Check sheet for the drawn part. Datum: minimum x, y, z corner. Units: mm. A direction names the side the tool comes from. Coordinates: 2 decimals unless noted, no trailing zeros. Order: outer loops, then holes, each group sorted by start corner. A loop starts at its lowest first (then second) coordinate and runs counter-clockwise, first axis right, second up. Notation, with made-up numbers: (73.5, -29) - (114.5, -29) arc R24 ccw to (114.5, -14) - close; hole circle Ø3 at (53.5, 34.5). An arc over 180 degrees is marked (long way). Return JSON: item names as keys, results as strings. Group by question number.
Item 1: Section check D-D on z = 38.5. Enter the section's corners in (x, y), then the cut area to 3 significant figures.
Item 2: Scan lines: probe 1 along Z at (x, y) = (3, 16.25); probe 2 along Y at (x, z) = (13, 127.5); probe 3 along X at (y, z) = (8.75, 122). Record each from-to range of solid material in increasing order.
Item 3: Section check C-C on z = 147. Enter the section's corners in (x, y).
Item 4: Tool access check on the marked faces 1, 2 and 3. Record the directions out of +Z, -Z, +X, -X, +Y, -Y that give a thin tool (end or side, any length) a straight path to the whole face; none if there is none.
Item 5: Section check A-A on x = 13. Enter the section's corners in (y, z).
Item 6: Gauge pin test, flat ends, axial feed: pin 1 (8 mm diameter, centred on x = 6, z = 137, fed in from -Y); pin 2 (12 mm diameter, centred on x = 11, z = 179.5, fed in from -Y); pin 3 (3 mm diameter, centred on x = 7, z = 144, fed in from +Y). Record the tip position at first contact, or that the pin passes through.
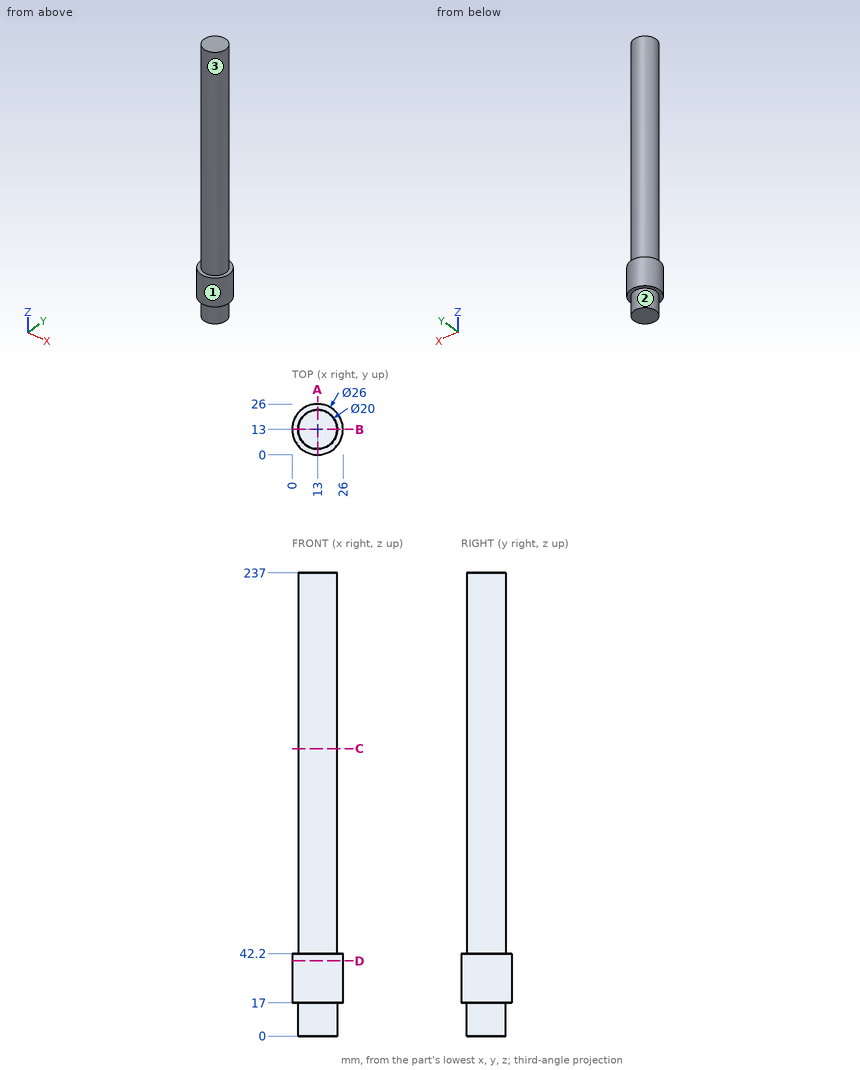
Computed:
{
 "1": {"outline": "circle Ø26 at (13, 13)", "area": "531 mm²"},
 "2": {"probe 1": "z = 17 to 42.2", "probe 2": "y = 3 to 23", "probe 3": "x = 3.95 to 22.05"},
 "3": {"outline": "circle Ø20 at (13, 13)"},
 "4": {"face 1": "+Z, -Z", "face 2": "-Z", "face 3": "+Z"},
 "5": {"outline": "(0, 17) - (3, 17) - (3, 0) - (23, 0) - (23, 17) - (26, 17) - (26, 42.2) - (23, 42.2) - (23, 237) - (3, 237) - (3, 42.2) - (0, 42.2) - close"},
 "6": {"pin 1": "stops at y = 3.46", "pin 2": "stops at y = 3", "pin 3": "stops at y = 21.93"}
}
